Source: three-view drawing plus pictorial views. Frame: mm from the lowest corner of the part. Round coordinates to 2 decimals unless told otherwise and drop trailing zeros. Write each loop counter-clockwise with the first axis right and the second up, starting at its lowest first coordinate (ties: lowest second). Pieces come first, ordered by that corner, then holes. Notation, with made-up numbers: M 9,81 L 42,81 A21 cw 42,120 Z; hole C 7.5,25 d5. An arc over 180 degrees is marked long. Answer as CSV lines item,"result". Start each with the question number.
Q1. Mould query, pull axis Y, two halves, no side actions, for the marked faces 1, 2 and 3. Classes: pulls with the +Y half, pulls with the -Y half, needs draft (parallel to the pull), parting line crosses it, or undercut.
Q2. Section query C-C on x = 41. Output: boundary loops of the cut face in (y, z), and give its area (3 significant figures).
Q3. Ray query, probe 1 along Y at (x, z) = (30, 9.25); probe 2 along Y at (x, z) = (55, 4.25); probe 3 along X at (y, z) = (6, 12). Return the intervals inside material, ascending.
Q4. Section query A-A on y = 30. Output: boundary loops of the cut face in (x, z).
Q5. Section query B-B on z = 2. Output: boundary loops of the cut face in (x, y) (3 decimals).
Q6. Section query D-D on y = 55. Output: boundary loops of the cut face in (x, z).
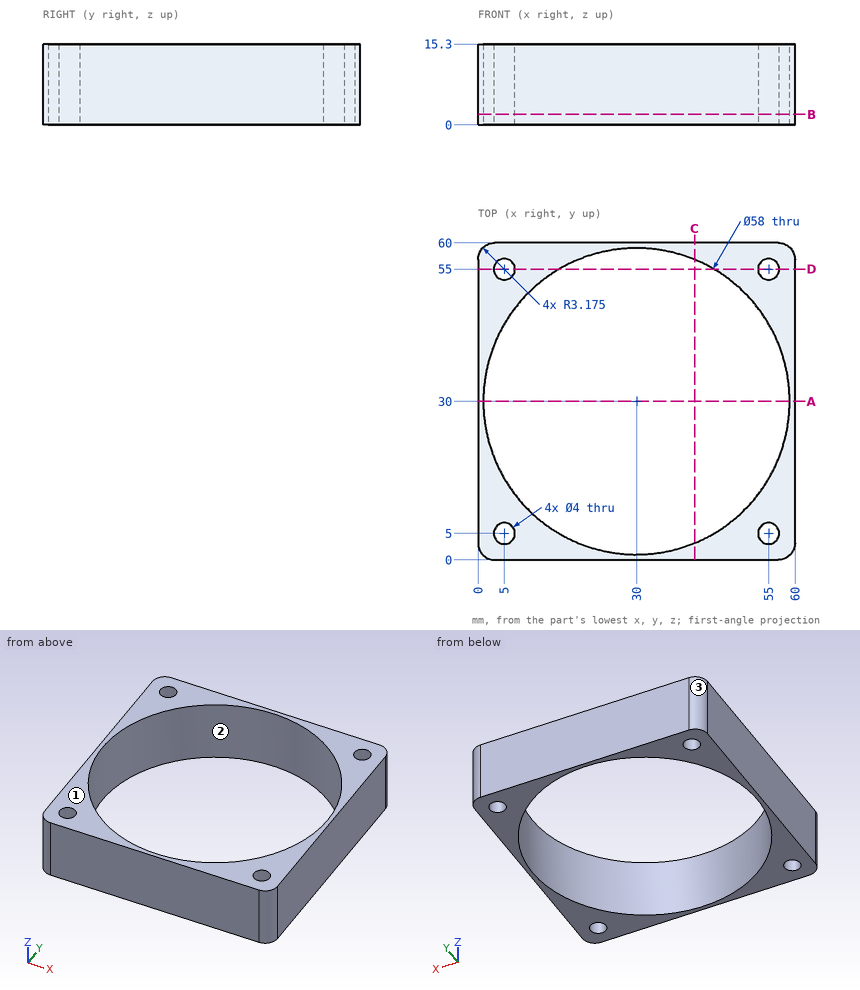
Entries:
1,face 1,"needs draft"
1,face 2,"undercut"
1,face 3,"pulls with the +Y half"
2,outline,"M 0,0 L 3.17,0 L 3.17,15.3 L 0,15.3 Z; M 56.83,0 L 60,0 L 60,15.3 L 56.83,15.3 Z"
2,area,"96.9 mm^2"
3,probe 1,"y = 0 to 1, 59 to 60"
3,probe 2,"y = 0 to 3, 7 to 15.3, 44.7 to 53, 57 to 60"
3,probe 3,"x = 0 to 3.27, 6.73 to 13.72, 46.28 to 53.27, 56.73 to 60"
4,outline,"M 0,0 L 1,0 L 1,15.3 L 0,15.3 Z; M 59,0 L 60,0 L 60,15.3 L 59,15.3 Z"
5,outline,"M 0,3.175 A3.175 ccw 3.175,0 L 56.825,0 A3.175 ccw 60,3.175 L 60,56.825 A3.175 ccw 56.825,60 L 3.175,60 A3.175 ccw 0,56.825 Z; hole C 30,30 d58; hole C 5,5 d4; hole C 5,55 d4; hole C 55,5 d4; hole C 55,55 d4"
6,outline,"M 0,0 L 3,0 L 3,15.3 L 0,15.3 Z; M 7,0 L 15.3,0 L 15.3,15.3 L 7,15.3 Z; M 44.7,0 L 53,0 L 53,15.3 L 44.7,15.3 Z; M 57,0 L 60,0 L 60,15.3 L 57,15.3 Z"
